Autodesk Inventor part; units mm, degrees
ref_plane "YZ Plane" through (0, 0, 0) normal (1, 0, 0) x (0, 1, 0)
ref_plane "XZ Plane" through (0, 0, 0) normal (0, 1, 0) x (-1, 0, 0)
ref_plane "XY Plane" through (0, 0, 0) normal (0, 0, 1) x (1, 0, 0)
sketch "스케치1" plane through (0, 0, 0) normal (0, 1, 0) x (-1, 0, 0)
  line L0 (-10.9012, 33.5504) -> (10.9012, 33.5504)
  line L1 (10.9012, 33.5504) -> (28.5397, 20.7353)
  line L2 (28.5397, 20.7353) -> (35.277, 0)
  line L3 (35.277, 0) -> (28.5397, -20.7353)
  line L4 (28.5397, -20.7353) -> (10.9012, -33.5504)
  line L5 (10.9012, -33.5504) -> (-10.9012, -33.5504)
  line L6 (-10.9012, -33.5504) -> (-28.5397, -20.7353)
  line L7 (-28.5397, -20.7353) -> (-35.277, 0)
  line L8 (-35.277, 0) -> (-28.5397, 20.7353)
  line L9 (-28.5397, 20.7353) -> (-10.9012, 33.5504)
  line L10 (11.9409, -36.7504) -> (-11.9409, -36.7504)
  line L11 (-11.9409, -36.7504) -> (-31.2618, -22.713)
  line L12 (-31.2618, -22.713) -> (-38.6417, 0)
  line L13 (-38.6417, 0) -> (-31.2618, 22.713)
  line L14 (-31.2618, 22.713) -> (-11.9409, 36.7504)
  line L15 (-11.9409, 36.7504) -> (11.9409, 36.7504)
  line L16 (11.9409, 36.7504) -> (31.2618, 22.713)
  line L17 (31.2618, 22.713) -> (38.6417, 0)
  line L18 (38.6417, 0) -> (31.2618, -22.713)
  line L19 (31.2618, -22.713) -> (11.9409, -36.7504)
  point P0 (0, 0)
  point P1 (0, 0)
  point P2 (0, 0)
  dimension "d0" = 70.554
  dimension "d1" = 3.2
extrude "돌출1" add sketch "스케치1" along normal blind 3.7 contours L0 L1 L2 L3 L4 L5 L6 L7 L8 L9 | L10 L11 L12 L13 L14 L15 L16 L17 L18 L19
sketch "스케치2" plane through (0, 3.7, 0) normal (0, 1, 0) x (1, 0, 0)
  line L0 (-11.4211, 35.1504) -> (11.4211, 35.1504)
  line L1 (11.4211, 35.1504) -> (29.9007, 21.7242)
  line L2 (29.9007, 21.7242) -> (36.9593, 0)
  line L3 (36.9593, 0) -> (29.9007, -21.7242)
  line L4 (29.9007, -21.7242) -> (11.4211, -35.1504)
  line L5 (11.4211, -35.1504) -> (-11.4211, -35.1504)
  line L6 (-11.4211, -35.1504) -> (-29.9007, -21.7242)
  line L7 (-29.9007, -21.7242) -> (-36.9593, 0)
  line L8 (-36.9593, 0) -> (-29.9007, 21.7242)
  line L9 (-29.9007, 21.7242) -> (-11.4211, 35.1504)
  line L10 (-31.2618, 22.713) -> (-38.6417, 0)
  point P0 (0, 0)
  point P1 (0, 0)
  dimension "d4" = 1.6
extrude "돌출2" cut sketch "스케치2" against normal blind 1.2
sketch "스케치3" plane through (0, 2.5, 0) normal (0, 1, 0) x (1, 0, 0)
  line L0 (-10.7712, 33.1504) -> (10.7712, 33.1504)
  line L1 (10.7712, 33.1504) -> (28.1994, 20.4881)
  line L2 (28.1994, 20.4881) -> (34.8564, 0)
  line L3 (34.8564, 0) -> (28.1994, -20.4881)
  line L4 (28.1994, -20.4881) -> (10.7712, -33.1504)
  line L5 (10.7712, -33.1504) -> (-10.7712, -33.1504)
  line L6 (-10.7712, -33.1504) -> (-28.1994, -20.4881)
  line L7 (-28.1994, -20.4881) -> (-34.8564, 0)
  line L8 (-34.8564, 0) -> (-28.1994, 20.4881)
  line L9 (-28.1994, 20.4881) -> (-10.7712, 33.1504)
  line L10 (-29.9007, 21.7242) -> (-11.4211, 35.1504)
  point P0 (0, 0)
  point P1 (0, 0)
  dimension "d7" = 2
extrude "돌출3" add sketch "스케치3" along normal blind 0.6
fillet "모깎기1" radius 1.2 20 edges at (0, 3.7, 36.7504) (0, 0, 36.7504) (-21.6014, 3.7, 29.7317) (-21.6014, 0, 29.7317) (-34.9517, 3.7, 11.3565) (-34.9517, 3.7, -11.3565) (-21.6014, 3.7, -29.7317) (0, 3.7, -36.7504) (21.6014, 3.7, -29.7317) (34.9517, 3.7, -11.3565) (34.9517, 3.7, 11.3565) (21.6014, 3.7, 29.7317) (21.6014, 0, -29.7317) (0, 0, -36.7504) (-21.6014, 0, -29.7317) (-34.9517, 0, -11.3565) (-34.9517, 0, 11.3565) (34.9517, 0, -11.3565) (34.9517, 0, 11.3565) (21.6014, 0, 29.7317)
sketch "스케치10" plane through (0, 0, 0) normal (0, -1, 0) x (1, 0, 0)
  line L0 (10.3, 12.5) -> (15.3, 12.5)
  line L1 (15.3, 12.5) -> (15.3, -12.5)
  line L2 (15.3, -12.5) -> (10.3, -12.5)
  line L3 (10.3, -12.5) -> (10.3, 12.5)
  line L4 (10.3, 12.5) -> (15.3, -12.5) construction
  line L5 (15.3, 12.5) -> (10.3, -12.5) construction
  line L6 (0, 0) -> (0, -7.1527)
  line L7 (-10.3, 12.5) -> (-15.3, 12.5)
  line L8 (-15.3, 12.5) -> (-15.3, -12.5)
  line L9 (-15.3, -12.5) -> (-10.3, -12.5)
  line L10 (-10.3, -12.5) -> (-10.3, 12.5)
  line L11 (-10.3, 12.5) -> (-15.3, -12.5) construction
  line L12 (-15.3, 12.5) -> (-10.3, -12.5) construction
  point P0 (12.8, 0)
  point P1 (-12.8, 0)
  dimension "d50" = 5
  dimension "d51" = 25
  dimension "d52" = 10.3
extrude "돌출7" add sketch "스케치10" along normal blind 15
sketch "스케치11" plane through (15.3, 0, 12.5) normal (1, 0, 0) x (0, 0, -1)
  circle A0 centre (7.5, -7.5) radius 1.25
  line L0 (-9.4714, 0) -> (12.5, 0)
  line L1 (12.5, 1.2) -> (12.5, 2.5)
  line L2 (12.5, 0) -> (12.5, -3.4496)
  circle A1 centre (17.5, -7.5) radius 1.25
  point P0 (12.5, 1.85)
  dimension "d55" = 2.5
  dimension "d56" = 7.5
  dimension "d57" = 5
extrude "돌출8" cut sketch "스케치11" against normal up to surface (30.6 mm away)
equation "\"d38\" = 55deg"
properties part number "OV-PAM_n_10_bottom"
Part model, mm, in its own coordinate system. A direction names the side the tool comes from. Round coordinates to 2 decimals unless told otherwise and drop trailing zeros. Write each loop counter-clockwise with the first axis right and the second up, starting at its lowest first coordinate (ties: lowest second). Pieces come first, ordered by that corner, then holes. Notation, with made-up numbers: M 43.25,87 L 49.25,87 A15 ccw 49.25,108 Z; hole C 15.25,-11.75 d3. An arc over 180 degrees is marked long. Return JSON: item names as keys, results as strings. Group by question number.
(1) Which spindle directions (+Z, -Z, +X, -X, +Y, -Y) get a long thin tool onto all of the face, cutting with end or side? Do faces 4 (the face through (-20.79, 3.108, -28.343)), 5 (the face through (15.3, -7, 0)), 6 (the face through (-10.3, -7, 0)). Say none if no direction does.
(2) Saw through at D-D on z = -5. Count the separate pieces of the cut face and the enclosed holes in it, then the cut area to 3 significant figures.
(3) Pin check, flat tips, straight feed: pin 1 Ø10 at (x, y) = (21, -1) entering from -Z; pin 2 Ø4 at (y, z) = (-7.5, 5) entering from -X; pin 3 Ø5.5 at (x, y) = (13, -8) entering from +Z. Stop position of each tip, or through.
(4) Saw through at A-A on y = -12.75. Write the cut outline in (x, z), then the cut area to 3 significant figures.
(5) Saw through at B-B on y = -7.5. Write the cut outline in (x, z).
(6) Two-plate mould, pull along Z, no slides. Class faces 1 (the face through (-33.48, 3.11, -10.71)), 2 (the face through (-13, -7, 12.5)), 3 (the face through (21.5, 0.3, -29.3)): +Z half, -Z half, draft (parallel to the pull), parting line (faces both ways), or undercut.
(7) Saw through at C-C on x = 9. Write the cut outline in (y, z).
(8) Drill centre lines: probe 1 along Y at (x, z) = (-13, -5); probe 2 along X at (y, z) = (-7, -8.5); probe 3 along Y at (x, z) = (14, 14.5). Where is each one in solid material? Low to high.
Returned:
{
 "1": {"face 4": "+Y", "face 5": "+Z, -Z, +X, -Y", "face 6": "+Z, -Z, -Y"},
 "2": {"separate pieces": "3", "enclosed holes": "0", "area": "353 mm²"},
 "3": {"pin 1": "z = -33.48", "pin 2": "x = -15.3", "pin 3": "z = 12.5"},
 "4": {"outline": "M -15.3,-12.5 L -10.3,-12.5 L -10.3,12.5 L -15.3,12.5 Z; M 10.3,-12.5 L 15.3,-12.5 L 15.3,12.5 L 10.3,12.5 Z", "area": "250 mm²"},
 "5": {"outline": "M -15.3,-12.5 L -10.3,-12.5 L -10.3,-6.25 L -15.3,-6.25 Z; M -15.3,-3.75 L -10.3,-3.75 L -10.3,3.75 L -15.3,3.75 Z; M -15.3,6.25 L -10.3,6.25 L -10.3,12.5 L -15.3,12.5 Z; M 10.3,-12.5 L 15.3,-12.5 L 15.3,-6.25 L 10.3,-6.25 Z; M 10.3,-3.75 L 15.3,-3.75 L 15.3,3.75 L 10.3,3.75 Z; M 10.3,6.25 L 15.3,6.25 L 15.3,12.5 L 10.3,12.5 Z"},
 "6": {"face 1": "undercut", "face 2": "+Z half", "face 3": "-Z half"},
 "7": {"outline": "M 0,-35.55 A1.2 ccw 1.2,-36.75 L 2.5,-36.75 A1.2 ccw 3.7,-35.55 L 3.7,-35.15 L 2.5,-35.15 L 2.5,-33.15 L 3.1,-33.15 L 3.1,33.15 L 2.5,33.15 L 2.5,35.15 L 3.7,35.15 L 3.7,35.55 A1.2 ccw 2.5,36.75 L 1.2,36.75 A1.2 ccw 0,35.55 Z"},
 "8": {"probe 1": "-15 to -8.75, -6.25 to 3.1", "probe 2": "-15.3 to -10.3, 10.3 to 15.3", "probe 3": "0 to 3.1"}
}
